Verification items for the finished model (mm, model axes). A direction names the side the tool comes from. Round coordinates to 2 decimals unless told otherwise and drop trailing zeros. Write each loop counter-clockwise with the first axis right and the second up, starting at its lowest first coordinate (ties: lowest second). Pieces come first, ordered by that corner, then holes. Notation, with made-up numbers: M -9.75,52.25 L 48.25,52.25 A30 cw 48.25,85.25 Z; hole C 50.25,-15.75 d3. An arc over 180 degrees is marked long. Write each question's results on one line, items separated by ' | '.
from build123d import *

# Parameters (mm, degrees)
F1_R  = 22.225
F4_R  = 22.225
F0_R  = 20.6375
F3_R  = 20.6375
F9_R  = 10.16
F8_R  = 6.35
F16_R = 14.892743
F15_R = 12.360635
F19_R = 23.686473
F13_R = 20.620664


with BuildPart() as f5:
    # F1 (on Top) → F5 section 0
    with BuildSketch(Plane.XY):
        Circle(F1_R)
    # F4 (on offset) → F5 section 1
    with BuildSketch(Plane.XY.offset(12.7)):
        Circle(F4_R)
    loft()

    # F0 (on Top) → F6 section 0
    with BuildSketch(Plane.XY):
        Circle(F0_R)
    # F3 (on offset) → F6 section 1
    with BuildSketch(Plane.XY.offset(12.7)):
        Circle(F3_R)
    loft(mode=Mode.SUBTRACT)

    # F1 (on Top) → F10 section 0
    with BuildSketch(Plane.XY):
        Circle(F1_R)
    # F9 (on offset) → F10 section 1
    with BuildSketch(Plane.XY.offset(-17.78)):
        Circle(F9_R)
    loft()

    # F8 (on offset) → F11 section 0
    with BuildSketch(Plane.XY.offset(-17.78)):
        Circle(F8_R)
    # F0 (on Top) → F11 section 1
    with BuildSketch(Plane.XY):
        Circle(F0_R)
    loft(mode=Mode.SUBTRACT)

    # F16 (on offset) → F17 section 0
    with BuildSketch(Plane.XY.offset(-30.48)):
        Circle(F16_R)
    # F9 (on offset) → F17 section 1
    with BuildSketch(Plane.XY.offset(-17.78)):
        Circle(F9_R)
    loft()

    # F15 (on offset) → F18 section 0
    with BuildSketch(Plane.XY.offset(-30.48)):
        Circle(F15_R)
    # F8 (on offset) → F18 section 1
    with BuildSketch(Plane.XY.offset(-17.78)):
        Circle(F8_R)
    loft(mode=Mode.SUBTRACT)

    # F19 (on offset) → F20 section 0
    with BuildSketch(Plane.XY.offset(-68.58)):
        Circle(F19_R)
    # F16 (on offset) → F20 section 1
    with BuildSketch(Plane.XY.offset(-30.48)):
        Circle(F16_R)
    loft()

    # F15 (on offset) → F21 section 0
    with BuildSketch(Plane.XY.offset(-30.48)):
        Circle(F15_R)
    # F13 (on offset) → F21 section 1
    with BuildSketch(Plane.XY.offset(-68.58)):
        Circle(F13_R)
    loft(mode=Mode.SUBTRACT)


solid = f5.part
1) Draft check along Z on faces 1 (the conical face through (5, -9.7, -19.8)), 2 (the flat face through (6, -20, 12.7)), 3 (the conical face through (-12.404, -9.511, -45.563)). Enter one of: pulls with the +Z half, pulls with the -Z half, needs draft (parallel to the pull), parting line crosses it, or undercut.
Calculated:
face 1: undercut | face 2: pulls with the +Z half | face 3: pulls with the -Z half
2) Sectioned sample at C-C, the plane z = -10. Record the cut outline in (x, y), and give its area (3 significant figures).
Calculated:
outline: C 0,0 d30.88; hole C 0,0 d25.2 | area: 250 mm²
3) Material ranges on line 1 (Y direction, x = 0, z = 2.75) (1 decimal); line 2 (X direction, y = -9.5, z = -58.5); line 3 (Y direction, x = 1, z = -46), recorded low to high. Write a range as [from, to].
Calculated:
line 1: y = [-22.2, -20.6], [20.6, 22.2] | line 2: x = [-19.13, -15.8], [15.8, 19.13] | line 3: y = [-18.45, -15.69], [15.69, 18.45]
4) Depth check by flat-ended pin: P1, Ø1.5, axis at x = 11.5, z = -28, coming from the -Y side; P2, Ø8, axis at x = -4, z = -30.5, coming from the -Y side; P3, Ø8, axis at x = 7.5, y = 6.5, coming from the +Z side; P4, Ø6, axis at x = 18, y = -5, coming from the -Z side. Enter the tip coordinate at first touch or a pass-through.
Calculated:
P1: stops at y = -9.02 | P2: stops at y = -15.57 | P3: stops at z = -8.35 | P4: stops at z = -68.58
5) Access from +Z, -Z, +X, -X, +Y, -Y to the whole of each face (thin tool, end or side, straight path). Record for faces 4 (the cylindrical face through (-4.474, -20.147, 6.439)), 5 (the flat face through (2, 21, -68.58)), 6 (the conical face through (17.41, 5.48, -45.03)).
Calculated:
face 4: +Z | face 5: -Z, +X, -X, +Y, -Y | face 6: none
